Geometry: final body of the model. Coordinates: model frame, mm. Give positions to 0.01 mm unless a question says otherwise; leave off trailing zeros. Order: outer loops, then holes, each group sorted by start corner. A loop starts at its lowest first (then second) coordinate and runs counter-clockwise, first axis right, second up. Notation, with made-up numbers: (-24.75, 79.25) -> (-19.75, 79.25) arc R21 ccw to (-19.75, 113.25) -> close; hole circle Ø11 at (73.25, 14.5). An arc over 180 degrees is marked (long way). Write item = value, one per line.
```python
from build123d import *

# Parameters (mm, degrees)
BOSS_EXTRUDE1_DEPTH = 2.5


with BuildPart() as part:
    # Sketch1 → Boss-Extrude1 (new, symmetric)
    with BuildSketch(Plane(origin=(0, 0, 0), x_dir=(0, 0, -1), z_dir=(1, 0, 0))):
        with BuildLine():
            ThreePointArc((-138.434966494, 10.875), (-135.24177294, 5.848962219), (-134.125, 0))
            Line((-134.125, 0), (134.125, 0))
            ThreePointArc((134.125, 0), (135.24177294, 5.848962219), (138.434966494, 10.875))
            Line((138.434966494, 10.875), (90, 10.875))
            Line((90, 10.875), (90, 15.875))
            Line((90, 15.875), (70, 15.875))
            Line((70, 15.875), (70, 10.875))
            Line((70, 10.875), (-70, 10.875))
            Line((-70, 10.875), (-70, 15.875))
            Line((-70, 15.875), (-90, 15.875))
            Line((-90, 15.875), (-90, 10.875))
            Line((-90, 10.875), (-138.434966494, 10.875))
        make_face()
    extrude(amount=BOSS_EXTRUDE1_DEPTH, both=True)


solid = part.part
```
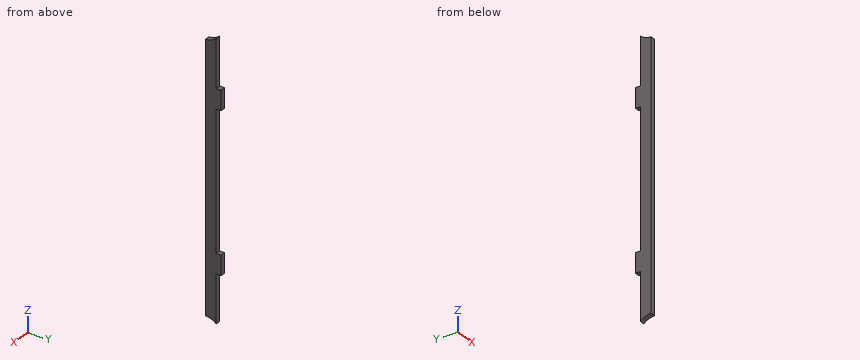
1) First-contact query: P1, Ø2.5, axis at x = -1, y = 13, coming from the -Z side; P2, Ø1.5, axis at x = -1, y = 12.5, coming from the +Z side; P3, Ø2, axis at x = -0.5, y = 3, coming from the +Z side. Flat tips, straight axial feed; report the tip coordinate or a pass-through.
Check sheet entries:
P1 = -90
P2 = 90
P3 = 134.64
2) Section query B-B (z = -96.5). Output: boundary loops of the cut face in (x, y) (3 decimals), plus the area to 3 significant figures.
Check sheet entries:
outline = (-2.5, 0) -> (2.5, 0) -> (2.5, 10.875) -> (-2.5, 10.875) -> close
area = 54.4 mm²
3) Section query A-A (x = -1.75). Output: boundary loops of the cut face in (y, z) (3 decimals), plus the area to 3 significant figures.
Check sheet entries:
outline = (0, -134.125) arc R15.875 cw to (10.875, -138.435) -> (10.875, -90) -> (15.875, -90) -> (15.875, -70) -> (10.875, -70) -> (10.875, 70) -> (15.875, 70) -> (15.875, 90) -> (10.875, 90) -> (10.875, 138.435) arc R15.875 cw to (0, 134.125) -> close
area = 3,150 mm²
4) Line query: line 1 (Z direction, x = 0, y = 13.5); line 2 (Y direction, x = -1.6, z = -13.5) (3 decimals); line 3 (Z direction, x = -0.15, y = 1.25). Output: solid intervals per line, ascending. Write a range as from..to.
Check sheet entries:
line_1 = -90..-70, 70..90
line_2 = 0..10.875
line_3 = -134.17..134.17
5) Section query C-C (y = 3). Output: boundary loops of the cut face in (x, z).
Check sheet entries:
outline = (-2.5, -134.41) -> (2.5, -134.41) -> (2.5, 134.41) -> (-2.5, 134.41) -> close
